from build123d import *

# Parameters (mm, degrees)
F0_W     = 6.5
F0_H     = 5.7
F1_DEPTH = 25
F2_DEPTH = 10
F3_SIZE  = 2
F5_D     = 3.5


with BuildPart() as f1:
    # F0 (on Top) → F1 (new body)
    with BuildSketch(Plane.XY):
        Polygon((2.5, 9), (-2.5, 9), (-2.5, 3.3), (-9, 3.3), (-9, -9), (9, -9), (9, 3.3), (2.5, 3.3), align=None)
        with Locations((-5.75, 6.15)):
            Rectangle(F0_W, F0_H)
        with Locations((5.75, 6.15)):
            Rectangle(F0_W, F0_H)
    extrude(amount=-F1_DEPTH)

    # F0 (on Top) → F2 (join)
    with BuildSketch(Plane.XY):
        Polygon((2.5, 9), (-2.5, 9), (-2.5, 3.3), (-9, 3.3), (-9, -9), (9, -9), (9, 3.3), (2.5, 3.3), align=None)
    extrude(amount=F2_DEPTH)

    # F3
    f3_edges = [f1.edges().sort_by_distance(p)[0] for p in [
        (0, 9, 10),
    ]]
    chamfer(f3_edges, length=F3_SIZE)

    # F5 (through all)
    with Locations(Plane.XZ.offset(9)):
        with Locations((-5, 6), (5, 6)):
            Hole(F5_D / 2)


solid = f1.part
The model under review builds one solid part; all positions refer to its coordinate system, in mm. A direction names the side the tool comes from. Round coordinates to 2 decimals unless told otherwise and drop trailing zeros. Order: outer loops, then holes, each group sorted by start corner. A loop starts at its lowest first (then second) coordinate and runs counter-clockwise, first axis right, second up. Notation, with made-up numbers: (-5.75, -6) -> (44.25, -6) arc R15 cw to (44.25, 19) -> close; hole circle Ø4 at (86.25, 31). An arc over 180 degrees is marked (long way). Use CSV: the item, a comma, the result in double quotes. Start each with the question number.
(1) Consider section A-A on z = 6. Write out the cut boundary in (x, y).
(2) Insertion check: pin 1 (3 mm diameter, centred on x = 5, z = 6, fed in from +Y); pin 2 (1.7 mm diameter, centred on x = -7, y = 7.5, fed in from +Z); pin 3 (1.7 mm diameter, centred on y = 6.5, z = 7, fed in from -X); pin 4 (5 mm diameter, centred on x = 7.5, z = 6.5, fed in from +Y). Each pin has a flat end and moves straight along its axis. Give the tip position at first contact, or say it passes through.
(3) Consider section B-B on x = 5. Write out the cut boundary in (y, z).
(4) Consider section C-C on y = -7.25. Write out the cut boundary in (x, z), and give its area (3 significant figures).
(5) Wall thickness on probe 1 along Z at (x, y) = (-5, -1.5); probe 2 along X at (y, z) = (-3, 7.5); probe 3 along Z at (x, y) = (-7.5, 6.75): over which ranges is each line inside the solid? List them lowest first. Write a range as from..to.
(6) Tool access review of faces 1 (the face through (2.5, 6, 5)), 2 (the face through (0, -3, 10)), 3 (the face through (-6, 3.3, 4)): name each direction out of +Z, -Z, +X, -X, +Y, -Y from which nothing blocks a thin tool from reaching the whole face with its end or side.
(7) Mouldability with a two-part tool opening along Z and no side actions: class faces 4 (the face through (5.38, -2.76, 4.29)), 5 (the face through (0, 8, 9)), 6 (the face through (9, 0, -7)) as pulls with the +Z half, pulls with the -Z half, needs draft (parallel to the pull), parting line crosses it, or undercut.
Responses:
1,outline,"(-9, -9) -> (-6.75, -9) -> (-6.75, 3.3) -> (-9, 3.3) -> close; (-3.25, -9) -> (3.25, -9) -> (3.25, 3.3) -> (2.5, 3.3) -> (2.5, 9) -> (-2.5, 9) -> (-2.5, 3.3) -> (-3.25, 3.3) -> close; (6.75, -9) -> (9, -9) -> (9, 3.3) -> (6.75, 3.3) -> close"
2,pin 1,"through"
2,pin 2,"z = 0"
2,pin 3,"x = -2.5"
2,pin 4,"y = 3.3"
3,outline,"(-9, -25) -> (9, -25) -> (9, 0) -> (3.3, 0) -> (3.3, 4.25) -> (-9, 4.25) -> close; (-9, 7.75) -> (3.3, 7.75) -> (3.3, 10) -> (-9, 10) -> close"
4,outline,"(-9, -25) -> (9, -25) -> (9, 10) -> (-9, 10) -> close; hole circle Ø3.5 at (-5, 6); hole circle Ø3.5 at (5, 6)"
4,area,"611 mm²"
5,probe 1,"-25..4.25, 7.75..10"
5,probe 2,"-9..-5.9, -4.1..4.1, 5.9..9"
5,probe 3,"-25..0"
6,face 1,"+Z, +X, +Y"
6,face 2,"+Z, +X, -X, +Y, -Y"
6,face 3,"+Z, -X, +Y"
7,face 4,"undercut"
7,face 5,"pulls with the +Z half"
7,face 6,"needs draft"
